Design review of the part built by this model. Coordinates are the model's own, in mm. Face numbers are marked on the shaded views. A direction names the side the tool comes from. Give positions to 0.01 mm unless a question says otherwise; leave off trailing zeros. Write each loop counter-clockwise with the first axis right and the second up, starting at its lowest first coordinate (ties: lowest second). Pieces come first, ordered by that corner, then holes.
Autodesk Inventor part; units mm, degrees
ref_plane "YZ Plane" through (0, 0, 0) normal (1, 0, 0) x (0, 1, 0)
ref_plane "XZ Plane" through (0, 0, 0) normal (0, 1, 0) x (-1, 0, 0)
ref_plane "XY Plane" through (0, 0, 0) normal (0, 0, 1) x (1, 0, 0)
sketch "Эскиз1" plane through (0, 0, 0) normal (0, 0, 1) x (1, 0, 0)
  circle A0 centre (-0.0141, -12.393) radius 25
  point P0 (0, 0)
  dimension "d0" = 50
extrude "Выдавливание1" add sketch "Эскиз1" along normal blind 30
sketch "Эскиз2" plane through (-0.0141, -12.393, 0) normal (0, 0, -1) x (-1, 0, 0)
  circle A0 centre (0, 0) radius 13.45
  point P0 (-0.0141, 12.393)
extrude "Выдавливание2" add sketch "Эскиз2" along normal blind 10
sketch "Эскиз3" plane through (-0.0141, -12.393, -10) normal (0, 0, -1) x (-1, 0, 0)
  circle A0 centre (0, 0) radius 8.5
  point P0 (-0.0141, 12.393)
  dimension "d5" = 17
extrude "Выдавливание3" add sketch "Эскиз3" along normal blind 10
sketch "Эскиз4" plane through (-0.0141, -12.393, -20) normal (0, 0, -1) x (-1, 0, 0)
  circle A0 centre (0, 0) radius 2.5
  point P0 (-0.0141, 12.393)
  dimension "d8" = 5
extrude "Выдавливание4" add sketch "Эскиз4" along normal blind 10
properties part number "Верх. часть штатива"
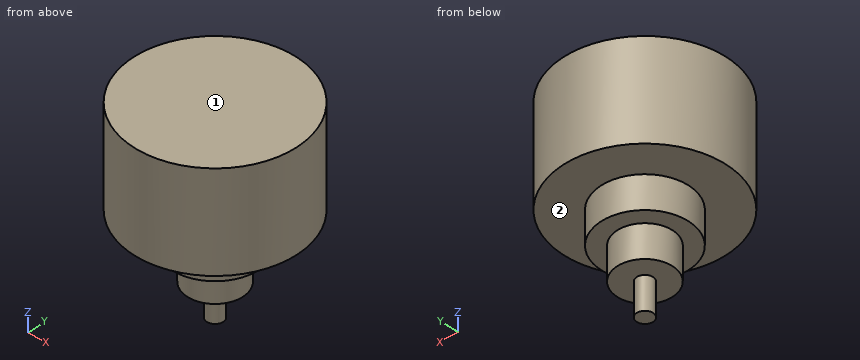
(1) Consider section A-A, the plane y = -23. Give the boundary of the cut face in (x, z).
Resolved:
outline: (-22.65, 0) - (-8.28, 0) - (-8.28, -10) - (8.26, -10) - (8.26, 0) - (22.62, 0) - (22.62, 30) - (-22.65, 30) - close
(2) Consider section B-B, the plane x = -7. Give the boundary of the cut face in (y, z).
Resolved:
outline: (-36.4, 0) - (-23.89, 0) - (-23.89, -10) - (-17.24, -10) - (-17.24, -20) - (-7.55, -20) - (-7.55, -10) - (-0.9, -10) - (-0.9, 0) - (11.61, 0) - (11.61, 30) - (-36.4, 30) - close
(3) Clearance check with flat-ended pins moving along their axes: P1, Ø2, axis at x = -10.5, y = -22.5, coming from the -Z side; P2, Ø3, axis at x = -1, z = 13.5, coming from the -Y side; P3, Ø15, axis at x = -6.5, y = -8, coming from the -Z side; P4, Ø12, axis at x = 13, z = 5.5, coming from the -Y side. State where each tip first meets the part, or that it passes through.
Resolved:
P1: stops at z = 0
P2: stops at y = -37.39
P3: stops at z = -30
P4: stops at y = -36.39
(4) Consider section D-D, the plane y = -7. Give the boundary of the cut face in (x, z).
Resolved:
outline: (-24.43, 0) - (-12.34, 0) - (-12.34, -10) - (-6.58, -10) - (-6.58, -20) - (6.56, -20) - (6.56, -10) - (12.31, -10) - (12.31, 0) - (24.4, 0) - (24.4, 30) - (-24.43, 30) - close
(5) Consider section C-C, the plane z = -13.5. Give the boundary of the cut face in (x, y).
Resolved:
outline: circle Ø17 at (-0.01, -12.39)
(6) Tool access review of the marked faces 1 and 2: name each direction out of +Z, -Z, +X, -X, +Y, -Y from which nothing blocks a thin tool from reaching the whole face with its end or side.
Resolved:
face 1: +Z, +X, -X, +Y, -Y
face 2: -Z
(7) To check wall thickness, follow L1, parallel to Z at x = -15, y = -3.5; L2, parallel to Z at x = 5.5, y = -18.5; L3, parallel to X at y = -12.5, z = -1. State the ranges of each line that lie inside material, in increasing order.
Resolved:
L1: z = 0 to 30
L2: z = -20 to 30
L3: x = -13.46 to 13.44
